The listing builds one solid part. Answer for the finished solid, in the listing's coordinates (mm). Face numbers are marked on the shaded views. A direction names the side the tool comes from. Coordinates: 2 decimals unless noted, no trailing zeros. Order: outer loops, then holes, each group sorted by start corner. A loop starts at its lowest first (then second) coordinate and runs counter-clockwise, first axis right, second up. Notation, with made-up numbers: (19.25, 40.25) - (28.25, 40.25) arc R17 ccw to (28.25, 54.25) - close; hole circle Ø8 at (39.25, -5). An arc over 180 degrees is marked (long way). Use a Markdown table: item, result. Add a question column.
Item 1: Find the intervals of material crossed by line 1 along Y through (x, z) = (2.75, 19.05) (3 decimals); line 2 along Z through (x, y) = (3.5, 9.25); line 3 along Z through (x, y) = (5.75, 2.5), in increasing order.
Item 2: The part is cut by section A-A, the plane z = 19.05. Give the vertices of the cut face in (x, y) (3 decimals).
Item 3: For the marked faces 5 and 6, determine the directions among +Z, -Z, +X, -X, +Y, -Y from which every point of the face is accessible in a straight line to the end or side of a thin tool.
Item 4: Flat-ended cylindrical pins translate along their axes: P1, Ø1.9, axis at x = 1.5, z = 4.5, coming from the -Y side; P2, Ø5.5, axis at y = 0, z = -19.05, coming from the +X side; P3, Ø1, axis at x = 2.5, z = -8.5, coming from the +Y side. Find the tip coordinate at first contact, or state that the pin passes through.
Item 5: The part is cut by section B-B, the plane y = 0. Give the vertices of the cut face in (x, z) (3 decimals), then the cut area to 3 significant figures.
Item 6: The part is cut by section C-C, the plane x = 4. Give the vertices of the cut face in (y, z) (3 decimals).
Item 7: The mould has two halves that part along Z. Classify the marked faces 1, 2, 3 and 4: released by +Z, released by -Z, zero draft, split by the parting line, or undercut.
Item 8: The part is cut by section D-D, the plane y = -7.5. Give the vertices of the cut face in (x, z).
from build123d import *

# Parameters (mm, degrees)
SKETCH1_R           = 3.175
BOSS_EXTRUDE1_DEPTH = 6.35


with BuildPart() as part:
    # Sketch1 → Boss-Extrude1 (new body)
    with BuildSketch(Plane(origin=(0, 0, 0), x_dir=(0, 0, -1), z_dir=(1, 0, 0))):
        Polygon((-20.32, 12.7), (-20.32, 6.35), (20.32, 6.35), (20.32, 12.7), (33.02, 12.7), (33.02, -12.7), (20.32, -12.7), (20.32, -6.35), (-20.32, -6.35), (-20.32, -12.7), (-33.02, -12.7), (-33.02, 12.7), align=None)
        with Locations((-19.05, 0)):
            Circle(SKETCH1_R, mode=Mode.SUBTRACT)
        with Locations((19.05, 0)):
            Circle(SKETCH1_R, mode=Mode.SUBTRACT)
    extrude(amount=BOSS_EXTRUDE1_DEPTH)


solid = part.part
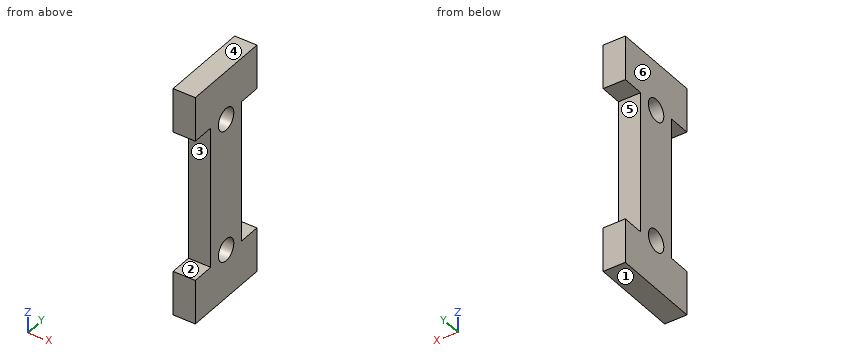
Solution:
| question | item | result |
|---|---|---|
| 1 | line 1 | y = -6.35 to -3.175, 3.175 to 6.35 |
| 1 | line 2 | z = -33.02 to -20.32, 20.32 to 33.02 |
| 1 | line 3 | z = -33.02 to -21.01, -17.09 to 17.09, 21.01 to 33.02 |
| 2 | outline | (0, -6.35) - (6.35, -6.35) - (6.35, -3.175) - (0, -3.175) - close; (0, 3.175) - (6.35, 3.175) - (6.35, 6.35) - (0, 6.35) - close |
| 3 | face 5 | +X, -X, +Y |
| 3 | face 6 | +Z, -Z, -X, +Y, -Y |
| 4 | P1 | stops at y = -6.35 |
| 4 | P2 | passes through |
| 4 | P3 | stops at y = 6.35 |
| 5 | outline | (0, -33.02) - (6.35, -33.02) - (6.35, -22.225) - (0, -22.225) - close; (0, -15.875) - (6.35, -15.875) - (6.35, 15.875) - (0, 15.875) - close; (0, 22.225) - (6.35, 22.225) - (6.35, 33.02) - (0, 33.02) - close |
| 5 | area | 339 mm2 |
| 6 | outline | (-12.7, -33.02) - (12.7, -33.02) - (12.7, -20.32) - (6.35, -20.32) - (6.35, 20.32) - (12.7, 20.32) - (12.7, 33.02) - (-12.7, 33.02) - (-12.7, 20.32) - (-6.35, 20.32) - (-6.35, -20.32) - (-12.7, -20.32) - close; hole circle Ø6.35 at (0, -19.05); hole circle Ø6.35 at (0, 19.05) |
| 7 | face 1 | released by -Z |
| 7 | face 2 | undercut |
| 7 | face 3 | undercut |
| 7 | face 4 | released by +Z |
| 8 | outline | (0, -33.02) - (6.35, -33.02) - (6.35, -20.32) - (0, -20.32) - close; (0, 20.32) - (6.35, 20.32) - (6.35, 33.02) - (0, 33.02) - close |
